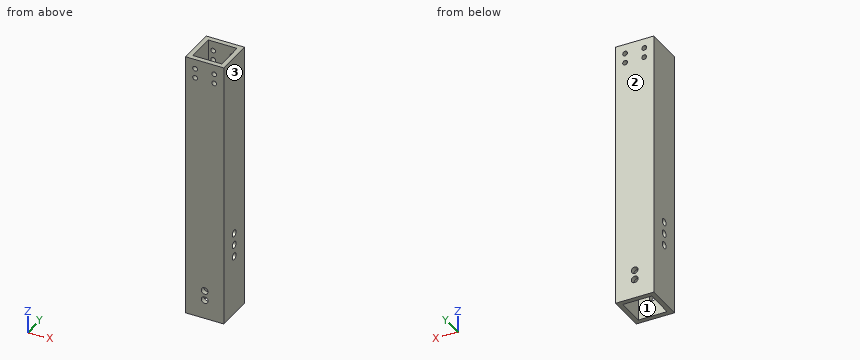
Autodesk Inventor part; units mm, degrees
ref_plane "YZ Plane" through (0, 0, 0) normal (1, 0, 0) x (0, 1, 0)
ref_plane "XZ Plane" through (0, 0, 0) normal (0, 1, 0) x (-1, 0, 0)
ref_plane "XY Plane" through (0, 0, 0) normal (0, 0, 1) x (1, 0, 0)
sketch "Sketch1" plane through (0, 0, 0) normal (0, 0, 1) x (1, 0, 0)
  line L0 (12.7, -12.7) -> (-12.7, -12.7)
  line L1 (-12.7, -12.7) -> (-12.7, 12.7)
  line L2 (-12.7, 12.7) -> (12.7, 12.7)
  line L3 (12.7, 12.7) -> (12.7, -12.7)
  line L4 (12.7, -12.7) -> (-12.7, 12.7) construction
  line L5 (-12.7, -12.7) -> (12.7, 12.7) construction
  line L6 (9.525, 9.525) -> (-9.525, 9.525)
  line L7 (-9.525, 9.525) -> (-9.525, -9.525)
  line L8 (-9.525, -9.525) -> (9.525, -9.525)
  line L9 (9.525, -9.525) -> (9.525, 9.525)
  point P0 (0, 0)
  dimension "d0" = 25.4
  dimension "d1" = 25.4
  dimension "d2" = 3.175
extrude "Extrusion1" add sketch "Sketch1" along normal blind 177.8
sketch "Sketch2" plane through (12.7, -12.7, 0) normal (1, 0, 0) x (0, 0, -1)
  line L0 (0, 0) -> (0, 25.4) construction
  line L1 (0, 25.4) -> (-177.8, 25.4) construction
  line L2 (-177.8, 0) -> (-177.8, 25.4) construction
  line L3 (0, 0) -> (-177.8, 0) construction
  line L4 (-177.8, 22.225) -> (-177.8, 3.175) construction
  line L5 (-177.8, 12.7) -> (0, 12.7) construction
  line L6 (-31.75, 25.4) -> (-31.75, 0) construction
  circle A0 centre (-39.75, 12.7) radius 2.25
  circle A1 centre (-47.75, 12.7) radius 2.25
  circle A2 centre (-55.75, 12.7) radius 2.25
  dimension "d5" = 31.75
  dimension "d6" = 4.5
  dimension "d7" = 8
  dimension "d8" = 4.5
  dimension "d9" = 8
  dimension "d10" = 4.5
  dimension "d11" = 8
extrude "Extrusion2" cut sketch "Sketch2" against normal through all
sketch "Sketch3" plane through (-12.7, 12.7, 0) normal (0, 1, 0) x (1, 0, 0)
  line L0 (12.7, 0) -> (12.7, -177.7213) construction
  circle A0 centre (12.7, -12.7) radius 2.25
  circle A1 centre (12.7, -19.05) radius 2.25
  line L1 (25.4, 0) -> (0, 0)
  dimension "d14" = 4.5
  dimension "d15" = 4.5
  dimension "d16" = 12.7
  dimension "d17" = 6.35
extrude "Extrusion3" cut sketch "Sketch3" against normal blind 25.4
sketch "Sketch4" plane through (-12.7, 12.7, 0) normal (0, 1, 0) x (1, 0, 0)
  line L0 (12.7, 0) -> (12.7, -177.8) construction
  line L1 (3.175, -177.8) -> (22.225, -177.8) construction
  circle A0 centre (6.35, -171.45) radius 1.5875
  line L2 (0, 0) -> (0, -177.8)
  circle A1 centre (19.05, -171.45) radius 1.5875
  line L3 (25.4, 0) -> (25.4, -177.8)
  circle A2 centre (6.35, -165.1) radius 1.5875
  circle A3 centre (19.05, -165.1) radius 1.5875
  dimension "d20" = 3.175
  dimension "d21" = 6.35
  dimension "d22" = 6.35
  dimension "d23" = 3.175
  dimension "d24" = 6.35
  dimension "d25" = 6.35
  dimension "d26" = 3.175
  dimension "d27" = 6.35
  dimension "d28" = 6.35
  dimension "d29" = 3.175
  dimension "d30" = 6.35
  dimension "d31" = 6.35
extrude "Extrusion4" cut sketch "Sketch4" against normal through all
properties part number "CS_Climb_Inner_Tube"
Here's how the part is built. I have some questions about the finished solid (model axes, mm). Face numbers are marked on the shaded views. Round coordinates to 2 decimals unless told otherwise and drop trailing zeros. Order: outer loops, then holes, each group sorted by start corner. A loop starts at its lowest first (then second) coordinate and runs counter-clockwise, first axis right, second up. Notation, with made-up numbers: M -0.5,22.5 L 27.5,22.5 A29 cw 27.5,44.5 Z; hole C 8.5,82 d1. An arc over 180 degrees is marked long. Return JSON: item names as keys, results as strings. Group by question number.
1. If we section it at C-C on y = 0: State how many separate pieces and enclosed holes the cut face has, then the cut area to 3 significant figures.
2. If we section it at B-B on z = 39.75: List the corners of the cut face in (x, y) for me (3 decimals).
3. Please list where these lines run through material, in increasing order: probe 1 along Z at (x, y) = (0, 10.4); probe 2 along Z at (x, y) = (-6.35, -11.3); probe 3 along X at (y, z) = (11.5, 165).
4. If we section it at D-D on y = 8: List the corners of the cut face in (x, z) for me (3 decimals), then the cut area to 3 significant figures.
5. I'm going to push a flat-ended pin straight in: pin 1 Ø6 at (x, y) = (-9.5, -9) entering from +Z. Where does the tip first touch, or does it pass through?
6. If we section it at A-A on x = 0: List the corners of the cut face in (y, z) for me (3 decimals).
7. If we mould it in two halves opening along Y, with no side actions, what happens to the marked faces 1, 2 and 3? For each: pulls with the +Y half, pulls with the -Y half, needs draft (parallel to the pull), parting line crosses it, or undercut.
Reply:
{
 "1": {"separate pieces": "8", "enclosed holes": "0", "area": "1,040 mm^2"},
 "2": {"outline": "M -12.7,-12.7 L 12.7,-12.7 L 12.7,-2.25 L 9.525,-2.25 L 9.525,-9.525 L -9.525,-9.525 L -9.525,-2.25 L -12.7,-2.25 Z; M -12.7,2.25 L -9.525,2.25 L -9.525,9.525 L 9.525,9.525 L 9.525,2.25 L 12.7,2.25 L 12.7,12.7 L -12.7,12.7 Z"},
 "3": {"probe 1": "0 to 10.45, 14.95 to 16.8, 21.3 to 177.8", "probe 2": "0 to 163.51, 166.69 to 169.86, 173.04 to 177.8", "probe 3": "-12.7 to -7.93, -4.77 to 4.77, 7.93 to 12.7"},
 "4": {"outline": "M -12.7,0 L -9.525,0 L -9.525,177.8 L -12.7,177.8 Z; M 9.525,0 L 12.7,0 L 12.7,177.8 L 9.525,177.8 Z", "area": "1,130 mm^2"},
 "5": {"pin 1": "z = 177.8"},
 "6": {"outline": "M -12.7,0 L -9.525,0 L -9.525,10.45 L -12.7,10.45 Z; M -12.7,14.95 L -9.525,14.95 L -9.525,16.8 L -12.7,16.8 Z; M -12.7,21.3 L -9.525,21.3 L -9.525,177.8 L -12.7,177.8 Z; M 9.525,0 L 12.7,0 L 12.7,10.45 L 9.525,10.45 Z; M 9.525,14.95 L 12.7,14.95 L 12.7,16.8 L 9.525,16.8 Z; M 9.525,21.3 L 12.7,21.3 L 12.7,177.8 L 9.525,177.8 Z"},
 "7": {"face 1": "undercut", "face 2": "pulls with the +Y half", "face 3": "needs draft"}
}
